```python
from build123d import *

# Parameters (mm, degrees)
ESQUISSE1_W             = 150
ESQUISSE1_H             = 200
BOSS_EXTRU_1_DEPTH      = 3
ESQUISSE2_W             = 150
ESQUISSE2_H             = 3
BOSS_EXTRU_2_DEPTH      = 80
ESQUISSE3_W             = 10
ESQUISSE3_H             = 10
ENL_V_MAT_EXTRU_1_DEPTH = 80
ESQUISSE4_R             = 0.75
BOSS_EXTRU_3_DEPTH      = 5
BOSS_EXTRU_5_START      = 5
ESQUISSE6_R             = 0.75
BOSS_EXTRU_5_DEPTH      = 5
ENL_V_MAT_EXTRU_2_DEPTH = 3
ESQUISSE10_W            = 60
ESQUISSE10_H            = 80
BOSS_EXTRU_9_DEPTH      = 3
ESQUISSE11_W            = 60
ESQUISSE11_H            = 80
BOSS_EXTRU_10_DEPTH     = 3
CONG_1_R                = 10


with BuildPart() as part:
    # Esquisse1 → Boss.-Extru.1 (new body)
    with BuildSketch(Plane.XY):
        with Locations((75, -100)):
            Rectangle(ESQUISSE1_W, ESQUISSE1_H)
    extrude(amount=BOSS_EXTRU_1_DEPTH)

    # Esquisse2 → Boss.-Extru.2 (add)
    with BuildSketch(Plane.XY.offset(3)):
        with Locations((75, -1.5)):
            Rectangle(ESQUISSE2_W, ESQUISSE2_H)
    extrude(amount=BOSS_EXTRU_2_DEPTH)

    # Esquisse3 → Enlèv. mat.-Extru.1 (cut)
    with BuildSketch(Plane(origin=(0, 0, 0), x_dir=(1, 0, 0), z_dir=(0, 1, 0))):
        with Locations((5, -78)):
            Rectangle(ESQUISSE3_W, ESQUISSE3_H)
        with Locations((145, -78)):
            Rectangle(ESQUISSE3_W, ESQUISSE3_H)
    extrude(amount=-ENL_V_MAT_EXTRU_1_DEPTH, mode=Mode.SUBTRACT)

    # Esquisse4 → Boss.-Extru.3 (add)
    with BuildSketch(Plane(origin=(140, 0, 0), x_dir=(0, 0, -1), z_dir=(1, 0, 0))):
        with Locations(Location((-78, -1.5, 0), (0, 0, 180))):
            Circle(ESQUISSE4_R)
    extrude(amount=BOSS_EXTRU_3_DEPTH)

    # Esquisse6 → Boss.-Extru.5 (add)
    with BuildSketch(Plane.ZY.offset(-10).offset(BOSS_EXTRU_5_START)):
        with Locations((78, -1.5)):
            Circle(ESQUISSE6_R)
    extrude(amount=-BOSS_EXTRU_5_DEPTH)

    # Esquisse9 → Enlèv. mat.-Extru.2 (cut)
    with BuildSketch(Plane(origin=(0, 0, 0), x_dir=(1, 0, 0), z_dir=(0, 1, 0))):
        with BuildLine():
            Line((41.1892956, -33.5), (0, -3))
            Line((0, -3), (0, -70))
            Line((0, -70), (41.1892956, -39.5))
            Line((41.1892956, -39.5), (57.361053438, -39.5))
            ThreePointArc((57.361053438, -39.5), (66.361053438, -36.5), (57.361053438, -33.5))
            Line((57.361053438, -33.5), (41.1892956, -33.5))
        make_face()
        with BuildLine():
            Line((150, -70), (150, -3))
            Line((150, -3), (108.8107044, -33.5))
            Line((108.8107044, -33.5), (92.638946562, -33.5))
            ThreePointArc((92.638946562, -33.5), (83.638946562, -36.5), (92.638946562, -39.5))
            Line((92.638946562, -39.5), (108.8107044, -39.5))
            Line((108.8107044, -39.5), (150, -70))
        make_face()
    extrude(amount=-ENL_V_MAT_EXTRU_2_DEPTH, mode=Mode.SUBTRACT)

    # Esquisse10 → Boss.-Extru.9 (add)
    with BuildSketch(Plane.ZY):
        with Locations((30, -130)):
            Rectangle(ESQUISSE10_W, ESQUISSE10_H)
    extrude(amount=BOSS_EXTRU_9_DEPTH)

    # Esquisse11 → Boss.-Extru.10 (add)
    with BuildSketch(Plane(origin=(150, 0, 0), x_dir=(0, 0, -1), z_dir=(1, 0, 0))):
        with Locations((-30, -130)):
            Rectangle(ESQUISSE11_W, ESQUISSE11_H)
    extrude(amount=BOSS_EXTRU_10_DEPTH)

    # Congé1
    cong_1_edges = [part.edges().sort_by_distance(p)[0] for p in [
        (-1.5, -170, 60),
        (-1.5, -90, 60),
        (151.5, -90, 60),
        (151.5, -170, 60),
    ]]
    fillet(cong_1_edges, radius=CONG_1_R)


solid = part.part
```
The model under review builds one solid part; all positions refer to its coordinate system, in mm. A direction names the side the tool comes from. Give positions to 0.01 mm unless a question says otherwise; leave off trailing zeros. Write each loop counter-clockwise with the first axis right and the second up, starting at its lowest first coordinate (ties: lowest second). Pieces come first, ordered by that corner, then holes.
(1) Tool access review of faces 1 (the flat face through (74, -100, 3)), 2 (the flat face through (129.69, -1.48, 18.04)), 3 (the flat face through (74, -3, 42)), 4 (the flat face through (20.31, -1.48, 54.96)), 5 (the flat face through (150, -129, 32)): name each direction out of +Z, -Z, +X, -X, +Y, -Y from which nothing blocks a thin tool from reaching the whole face with its end or side.
(2) For P1, Ø1.2, axis at y = -1.5, z = 78, coming from the +X side; P2, Ø8, axis at x = 25, y = -169, coming from the +Z side; P3, Ø4, axis at x = 28.5, z = 60.5, coming from the -Y side, all flat-tipped, find the tip position at first contact; note any pin that passes through.
(3) Consider section A-A, the plane z = 36.5. Give the boundary of the cut face in (x, y), and give its area (3 significant figures).
(4) Consider section C-C, the plane y = -77. Give the boundary of the cut face in (x, z), and give its area (3 significant figures).
(5) To check wall thickness, follow L1, parallel to Z at x = 76, y = -136.5; L2, parallel to Y at x = 59.5, z = 72; L3, parallel to X at y = -98, z = 13.5. State the ranges of each line that lie inside material, in increasing order.
(6) Consider section D-D, the plane z = 57.5. Give the boundary of the cut face in (x, y).
(7) Consider section B-B, the plane x = 34. Give the boundary of the cut face in (y, z), and give its area (3 significant figures).
(8) The part is to be moulded in two halves that separate along X. For faces 6 (the flat face through (74, -101, 0)), 7 (the flat face through (0, -129, 31)), 8 (the flat face through (20.88, -1.48, 18.46)), say which applies: released by +X, released by -X, zero draft, split by the parting line, or undercut.
Returned:
1. face 1: +Z, -Y
1. face 2: +X, +Y, -Y
1. face 3: +Z, +X, -X, -Y
1. face 4: -X, +Y, -Y
1. face 5: +Z, +Y, -Y
2. P1: stops at x = 145
2. P2: stops at z = 3
2. P3: stops at y = -3
3. outline: (-3, -170) - (0, -170) - (0, -90) - (-3, -90) - close; (66.36, -3) - (83.64, -3) - (83.64, 0) - (66.36, 0) - close; (150, -170) - (153, -170) - (153, -90) - (150, -90) - close
3. area: 532 mm2
4. outline: (0, 0) - (150, 0) - (150, 3) - (0, 3) - close
4. area: 450 mm2
5. L1: z = 0 to 3
5. L2: y = -3 to 0
5. L3: x = -3 to 0, 150 to 153
6. outline: (-3, -166.61) - (0, -166.61) - (0, -93.39) - (-3, -93.39) - close; (16.88, -3) - (133.12, -3) - (133.12, 0) - (16.88, 0) - close; (150, -166.61) - (153, -166.61) - (153, -93.39) - (150, -93.39) - close
7. outline: (-200, 0) - (0, 0) - (0, 28.18) - (-3, 28.18) - (-3, 3) - (-200, 3) - close; (-3, 44.82) - (0, 44.82) - (0, 83) - (-3, 83) - close
7. area: 790 mm2
8. face 6: zero draft
8. face 7: undercut
8. face 8: released by -X
